```python
from build123d import *

# Parameters (mm, degrees)
BOSS_EXTRUDE1_DEPTH            = 5
CBORE_FOR_M3_SHCS1_D           = 3.6
CBORE_FOR_M3_SHCS1_DEPTH       = 5
CBORE_FOR_M3_SHCS1_CBORE_D     = 6.5
CBORE_FOR_M3_SHCS1_CBORE_DEPTH = 3
CBORE_FOR_M3_SHCS1_TIP         = 1.081549114
FILLET1_R                      = 5


with BuildPart() as part:
    # Sketch1 → Boss-Extrude1 (new body, symmetric)
    with BuildSketch(Plane(origin=(0, 0, 0), x_dir=(0, 0, -1), z_dir=(1, 0, 0))):
        with BuildLine():
            Line((-32.5, 0), (-12.5, 0))
            ThreePointArc((-12.5, 0), (0, 12.5), (12.5, 0))
            Line((12.5, 0), (32.5, 0))
            Line((32.5, 0), (32.5, 5))
            Line((32.5, 5), (16.770509831, 5))
            ThreePointArc((16.770509831, 5), (0, 17.5), (-16.770509831, 5))
            Line((-16.770509831, 5), (-32.5, 5))
            Line((-32.5, 5), (-32.5, 0))
        make_face()
    extrude(amount=BOSS_EXTRUDE1_DEPTH, both=True)

    # CBORE for M3 SHCS1
    with Locations(Plane(origin=(-41.05, 5, 0), x_dir=(1, 0, 0), z_dir=(0, 1, 0))):
        with Locations((41.05, -27.5), (41.05, 27.5)):
            CounterBoreHole(CBORE_FOR_M3_SHCS1_D / 2, CBORE_FOR_M3_SHCS1_CBORE_D / 2, CBORE_FOR_M3_SHCS1_CBORE_DEPTH, depth=CBORE_FOR_M3_SHCS1_DEPTH)
            with Locations((0, 0, -(CBORE_FOR_M3_SHCS1_DEPTH + CBORE_FOR_M3_SHCS1_TIP / 2))):  # 118° drill point
                Cone(0, CBORE_FOR_M3_SHCS1_D / 2, CBORE_FOR_M3_SHCS1_TIP, mode=Mode.SUBTRACT)

    # Fillet1
    fillet1_edges = [part.edges().sort_by_distance(p)[0] for p in [
        (0, 5, 16.770509831),
        (0, 5, -16.770509831),
    ]]
    fillet(fillet1_edges, radius=FILLET1_R)


solid = part.part
```
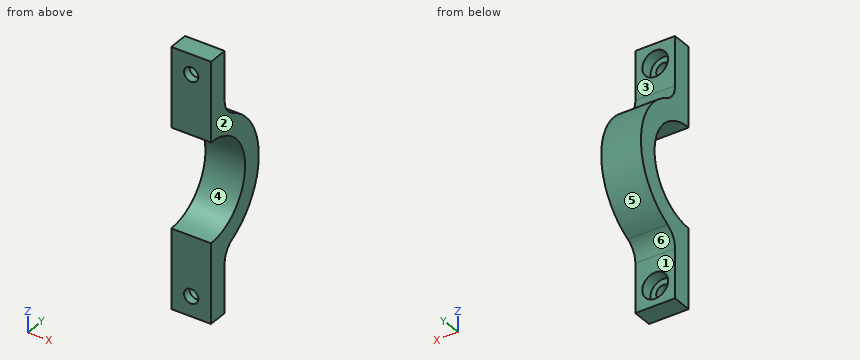
Build history of the part. All positions in model axes, mm. Face numbers are marked on the shaded views. A direction names the side the tool comes from. Coordinates: 2 decimals unless noted, no trailing zeros. Order: outer loops, then holes, each group sorted by start corner. A loop starts at its lowest first (then second) coordinate and runs counter-clockwise, first axis right, second up. Notation, with made-up numbers: M -28,-25 L -24,-25 A25 cw -24,-13 Z; hole C 43,21.25 d7. An arc over 180 degrees is marked long. One line per question, with ' | ' between items. Start each with the question number.
1. Mould opens along Z. For the marked faces 4, 5 and 6 say: +Z half, -Z half, draft (parallel to the pull), parting line (faces both ways), or undercut.
2. Cut at A-A (x = 0). Write the cut outline in (y, z), plus the area to 3 significant figures.
3. Cut at B-B (z = 27.5). Write the cut outline in (x, y), plus the area to 3 significant figures.
4. Wall check: line 1 along Z through (x, y) = (0, 2.75); line 2 along X through (y, z) = (0.85, -27.5); line 3 along Z through (x, y) = (1.25, 4.25). Give the ranges that are in metal, low to high. Write a range as [from, to].
5. Cut at C-C (y = 6). Write the cut outline in (x, z), plus the area to 3 significant figures.
6. Tool access for the marked faces 1, 2 and 3: list every direction of +Z, -Z, +X, -X, +Y, -Y with a clear straight run to the whole face (end or side of a thin tool).
7. Flat gauge pins, fed straight in: P1, Ø10, axis at y = 11, z = 26, coming from the +X side; P2, Ø4.5, axis at x = 0, z = -27.5, coming from the +Y side; P3, Ø5, axis at x = -1, z = 29, coming from the +Y side. Where does each tip first touch, or does it go through?
8. Cut at D-D (y = 11.75). Write the cut outline in (x, z).
The answers:
1) face 4: undercut | face 5: parting line | face 6: -Z half
2) outline: M 0,-32.5 L 5,-32.5 L 5,-30.75 L 2,-30.75 L 2,-29.3 L 0,-29.3 Z; M 0,-25.7 L 2,-25.7 L 2,-24.25 L 5,-24.25 L 5,-20.16 A5 cw 7.78,-15.68 A17.5 ccw 7.78,15.68 A5 cw 5,20.16 L 5,24.25 L 2,24.25 L 2,25.7 L 0,25.7 L 0,12.5 A12.5 cw 0,-12.5 Z; M 0,29.3 L 2,29.3 L 2,30.75 L 5,30.75 L 5,32.5 L 0,32.5 Z | area: 338 mm2
3) outline: M -5,0 L -1.8,0 L -1.8,2 L -3.25,2 L -3.25,5 L -5,5 Z; M 1.8,0 L 5,0 L 5,5 L 3.25,5 L 3.25,2 L 1.8,2 Z | area: 23.3 mm2
4) line 1: z = [-32.5, -30.75], [-24.25, -12.19], [12.19, 24.25], [30.75, 32.5] | line 2: x = [-5, -1.8], [1.8, 5] | line 3: z = [-32.5, -30.5], [-24.5, -11.76], [11.76, 24.5], [30.5, 32.5]
5) outline: M -5,-17.16 L 5,-17.16 L 5,-10.97 L -5,-10.97 Z; M -5,10.97 L 5,10.97 L 5,17.16 L -5,17.16 Z | area: 124 mm2
6) face 1: -Z, +X, -X, +Y | face 2: +Z, -Z, +X, +Y, -Y | face 3: +Z, +X, -X, +Y
7) P1: passes through | P2: stops at y = 2 | P3: stops at y = 5
8) outline: M -5,-12.97 L 5,-12.97 L 5,-4.26 L -5,-4.26 Z; M -5,4.26 L 5,4.26 L 5,12.97 L -5,12.97 Z
